Build history of the part. All positions in model axes, mm. Give positions to 0.01 mm unless a question says otherwise; leave off trailing zeros. Use a Markdown table: item, result. Add a question column.
```python
from build123d import *

# Parameters (mm, degrees)
SZKIC1_W                    = 185
SZKIC1_H                    = 69
DODANIE_WYCI_GNI_CIE1_DEPTH = 6
WYTNIJ_WYCI_GNI_CIE2_DEPTH  = 203.495320778
SZYK_LINIOWY1_COUNT         = 2
SZYK_LINIOWY1_PITCH         = 90
WYTNIJ_WYCI_GNI_CIE3_DEPTH  = 203.495320778
SZYK_LINIOWY2_COUNT         = 2
SZYK_LINIOWY2_PITCH         = 28.9
SZKIC8_R                    = 1.55
WYTNIJ_WYCI_GNI_CIE4_DEPTH  = 203.495320778
SZKIC11_R                   = 2.05
SZKIC11_R_2                 = 1.55
WYTNIJ_WYCI_GNI_CIE7_DEPTH  = 10
SZKIC13_R                   = 1.55
WYTNIJ_WYCI_GNI_CIE8_DEPTH  = 6
SZKIC14_W                   = 7
SZKIC14_H                   = 1.5
WYTNIJ_WYCI_GNI_CIE9_DEPTH  = 10
SZKIC16_R                   = 1.55
WYTNIJ_WYCI_GNI_CIE10_DEPTH = 6


with BuildPart() as part:
    # Szkic1 → Dodanie-wyciągnięcie1 (new body)
    with BuildSketch(Plane.XY):
        with Locations((-82.8, 66.684311715)):
            Rectangle(SZKIC1_W, SZKIC1_H)
    extrude(amount=-DODANIE_WYCI_GNI_CIE1_DEPTH)

    # Szkic6 → Wytnij-wyciągnięcie2 (cut, through all)
    with BuildSketch(Plane(origin=(0, 0, -6), x_dir=(-1, 0, 0), z_dir=(0, 0, -1))):
        Polygon((135.3, 101.184311715), (132.2, 101.184311715), (132.2, 97.184311715), (130.825, 97.184311715), (130.825, 95.184311715), (132.2, 95.184311715), (132.2, 94.684311715), (135.3, 94.684311715), (135.3, 95.184311715), (136.675, 95.184311715), (136.675, 97.184311715), (135.3, 97.184311715), align=None)
    wytnij_wyci_gni_cie2 = extrude(amount=-WYTNIJ_WYCI_GNI_CIE2_DEPTH, mode=Mode.SUBTRACT)

    # Szyk liniowy1: Wytnij-wyciągnięcie2 ×2
    with Locations(*[(i * SZYK_LINIOWY1_PITCH, 0, 0) for i in range(1, SZYK_LINIOWY1_COUNT)]):
        add(wytnij_wyci_gni_cie2, mode=Mode.SUBTRACT)

    # Szkic7 → Wytnij-wyciągnięcie3 (cut, through all)
    with BuildSketch(Plane(origin=(0, 0, -6), x_dir=(-1, 0, 0), z_dir=(0, 0, -1))):
        Polygon((-9.7, 86.184311715), (-9.7, 83.084311715), (-5.7, 83.084311715), (-5.7, 81.709311715), (-3.7, 81.709311715), (-3.7, 83.084311715), (-3.2, 83.084311715), (-3.2, 86.184311715), (-3.7, 86.184311715), (-3.7, 87.559311715), (-5.7, 87.559311715), (-5.7, 86.184311715), align=None)
    wytnij_wyci_gni_cie3 = extrude(amount=-WYTNIJ_WYCI_GNI_CIE3_DEPTH, mode=Mode.SUBTRACT)

    # Szyk liniowy2: Wytnij-wyciągnięcie3 ×2
    with Locations(*[(0, -i * SZYK_LINIOWY2_PITCH, 0) for i in range(1, SZYK_LINIOWY2_COUNT)]):
        add(wytnij_wyci_gni_cie3, mode=Mode.SUBTRACT)

    # Szkic8 → Wytnij-wyciągnięcie4 (cut, through all)
    with BuildSketch(Plane(origin=(0, 0, -6), x_dir=(-1, 0, 0), z_dir=(0, 0, -1))):
        with Locations((111.3, 96.184311715)):
            Circle(SZKIC8_R)
        with Locations((111.3, 64.184311715)):
            Circle(SZKIC8_R)
        with Locations((3.3, 64.184311715)):
            Circle(SZKIC8_R)
        with Locations((3.3, 96.184311715)):
            Circle(SZKIC8_R)
    extrude(amount=-WYTNIJ_WYCI_GNI_CIE4_DEPTH, mode=Mode.SUBTRACT)

    # Szkic11 → Wytnij-wyciągnięcie7 (cut)
    with BuildSketch(Plane(origin=(0, 0, -6), x_dir=(-1, 0, 0), z_dir=(0, 0, -1))):
        with Locations((170.3, 97.184311715)):
            Circle(SZKIC11_R)
        with Locations((152.3, 97.184311715)):
            Circle(SZKIC11_R_2)
        with Locations((126.3, 97.184311715)):
            Circle(SZKIC11_R_2)
    extrude(amount=-WYTNIJ_WYCI_GNI_CIE7_DEPTH, mode=Mode.SUBTRACT)

    # Szkic13 → Wytnij-wyciągnięcie8 (cut)
    with BuildSketch(Plane(origin=(0, 0, -6), x_dir=(-1, 0, 0), z_dir=(0, 0, -1))):
        with Locations((49.977029411, 45.18796276)):
            Circle(SZKIC13_R)
        with Locations((50.06, 55.184311715)):
            Circle(SZKIC13_R)
        with Locations((0.54, 55.184311715)):
            Circle(SZKIC13_R)
        with Locations((0.622970589, 45.18796276)):
            Circle(SZKIC13_R)
        with BuildLine():
            Line((6.3, 39.884311715), (44.3, 39.884311715))
            ThreePointArc((44.3, 39.884311715), (45.219238816, 40.265072899), (45.6, 41.184311715))
            Line((45.6, 41.184311715), (45.6, 59.184311715))
            ThreePointArc((45.6, 59.184311715), (45.219238816, 60.10355053), (44.3, 60.484311715))
            Line((44.3, 60.484311715), (6.3, 60.484311715))
            ThreePointArc((6.3, 60.484311715), (5.380761184, 60.10355053), (5, 59.184311715))
            Line((5, 59.184311715), (5, 41.184311715))
            ThreePointArc((5, 41.184311715), (5.380761184, 40.265072899), (6.3, 39.884311715))
        make_face()
    extrude(amount=-WYTNIJ_WYCI_GNI_CIE8_DEPTH, mode=Mode.SUBTRACT)

    # Szkic14 → Wytnij-wyciągnięcie9 (cut)
    with BuildSketch(Plane(origin=(0, 0, -6), x_dir=(-1, 0, 0), z_dir=(0, 0, -1))):
        with Locations((49.1, 50.184311715)):
            Rectangle(SZKIC14_W, SZKIC14_H)
        with Locations((1.5, 50.184311715)):
            Rectangle(SZKIC14_W, SZKIC14_H)
    extrude(amount=-WYTNIJ_WYCI_GNI_CIE9_DEPTH, mode=Mode.SUBTRACT)

    # Szkic16 → Wytnij-wyciągnięcie10 (cut)
    with BuildSketch(Plane(origin=(0, 0, -6), x_dir=(-1, 0, 0), z_dir=(0, 0, -1))):
        with Locations((153.3, 89.734311715)):
            Circle(SZKIC16_R)
        with Locations((153.3, 71.734311715)):
            Circle(SZKIC16_R)
    extrude(amount=-WYTNIJ_WYCI_GNI_CIE10_DEPTH, mode=Mode.SUBTRACT)


solid = part.part
```
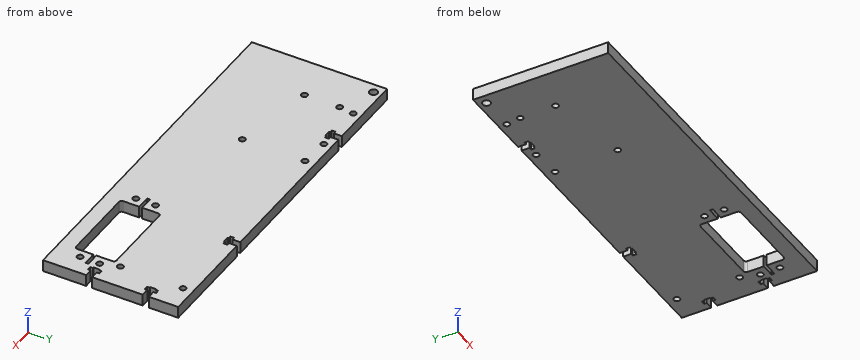
(1) Pin check, flat tips, straight feed: pin 1 Ø5 at (x, y) = (-3.3, 96.18) entering from -Z; pin 2 Ø2.5 at (x, y) = (-111.3, 64.18) entering from +Z. Stop position of each tip, or through.
(2) Band-saw the part on A-A on z = -4.2. State how many separate pieces and enclosed holes the cut face has, plus the area to 3 significant figures.
(3) Wall check: probe 1 along Y at (x, z) = (-3.3, -4.3); probe 2 along Y at (x, z) = (-0.54, -2.05); probe 3 along Y at (x, z) = (-29, -2.65). Give the ranges that are in metal, low to high.
Response:
| question | item | result |
|---|---|---|
| 1 | pin 1 | stops at z = -6 |
| 1 | pin 2 | passes through |
| 2 | separate pieces | 1 |
| 2 | enclosed holes | 14 |
| 2 | area | 11,700 mm² |
| 3 | probe 1 | y = 32.18 to 49.43, 50.93 to 62.63, 65.73 to 94.63, 97.73 to 101.18 |
| 3 | probe 2 | y = 32.18 to 43.64, 46.74 to 49.43, 50.93 to 53.63, 56.73 to 101.18 |
| 3 | probe 3 | y = 32.18 to 39.88, 60.48 to 101.18 |
